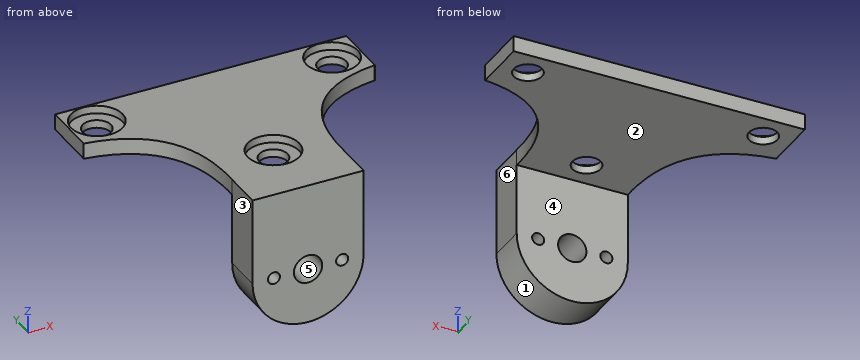
from build123d import *

# Parameters (mm, degrees)
ESQUISSE1_R             = 3.575
BOSS_EXTRU_1_DEPTH      = 4
ESQUISSE17_R            = 6.5
ENL_V_MAT_EXTRU_9_DEPTH = 2
ESQUISSE18_R            = 3.575
ESQUISSE18_R_2          = 1.525
BOSS_EXTRU_6_DEPTH      = 10


with BuildPart() as part:
    # Esquisse1 → Boss.-Extru.1 (new body)
    with BuildSketch(Plane.XY):
        with BuildLine():
            Line((0, 42.932447878), (0, 28.932447878))
            add(Edge.make_bspline(
                [(0, 28.932447878), (23.217449625, 26.022104371), (22.625, 0)],
                knots=[0, 0, 0, 1, 1, 1], degree=2))
            Line((22.625, 0), (36.625, 0))
            Line((36.625, 0), (50.625, 0))
            add(Edge.make_bspline(
                [(73.25, 28.932447878), (50.032550375, 26.022104371), (50.625, 0)],
                knots=[0, 0, 0, 1, 1, 1], degree=2))
            Line((73.25, 28.932447878), (73.4, 28.932447878))
            Line((73.4, 28.932447878), (73.4, 42.932447878))
            Line((73.4, 42.932447878), (0, 42.932447878))
        make_face()
        with Locations((7.025, 36.178525203)):
            Circle(ESQUISSE1_R, mode=Mode.SUBTRACT)
        with Locations((66.375, 36.245920154)):
            Circle(ESQUISSE1_R, mode=Mode.SUBTRACT)
        with Locations((36.625, 7.025)):
            Circle(ESQUISSE1_R, mode=Mode.SUBTRACT)
    extrude(amount=BOSS_EXTRU_1_DEPTH)

    # Esquisse17 → Enlèv. mat.-Extru.9 (cut)
    with BuildSketch(Plane.XY.offset(4)):
        with Locations((7.025, 36.178525203)):
            Circle(ESQUISSE17_R)
        with Locations((66.375, 36.245920154)):
            Circle(ESQUISSE17_R)
        with Locations((36.625, 7.025)):
            Circle(ESQUISSE17_R)
    extrude(amount=-ENL_V_MAT_EXTRU_9_DEPTH, mode=Mode.SUBTRACT)

    # Esquisse18 → Boss.-Extru.6 (add)
    with BuildSketch(Plane.XZ):
        with BuildLine():
            Line((22.625, -18), (22.625, 4))
            Line((22.625, 4), (50.625, 4))
            Line((50.625, 4), (50.625, -18))
            ThreePointArc((50.625, -18), (36.625, -32), (22.625, -18))
        make_face()
        with Locations((36.625, -18)):
            Circle(ESQUISSE18_R, mode=Mode.SUBTRACT)
        with Locations((28.025, -18)):
            Circle(ESQUISSE18_R_2, mode=Mode.SUBTRACT)
        with Locations((45.225, -18)):
            Circle(ESQUISSE18_R_2, mode=Mode.SUBTRACT)
    extrude(amount=BOSS_EXTRU_6_DEPTH)


solid = part.part
Work out the finished part from the listing and answer in its coordinate system (mm). Face numbers are marked on the shaded views. A direction names the side the tool comes from. Round coordinates to 2 decimals unless told otherwise and drop trailing zeros. Write each loop counter-clockwise with the first axis right and the second up, starting at its lowest first coordinate (ties: lowest second). Pieces come first, ordered by that corner, then holes. Notation, with made-up numbers: (30.25, 45.25) - (56.25, 45.25) arc R9 ccw to (56.25, 50.25) - close; hole circle Ø7 at (-3.75, 48.5). An arc over 180 degrees is marked (long way). Answer in a Markdown table with one row per item. Add a question column.
1. Find the intervals of material crossed by line 1 along Z through (x, y) = (63, 27); line 2 along Y through (x, z) = (38, -29); line 3 along X through (y, z) = (-2.5, -18.5), in increasing order. Write a range as from..to.
2. A cutting plane is placed at C-C, the plane z = -1. Determine the outline of the cut face in (x, y) (3 decimals), and give its area (3 significant figures).
3. A cutting plane is placed at A-A, the plane y = 35. Determine the outline of the cut face in (x, z), and give its area (3 significant figures).
4. The mould has two halves that part along X. Classify the marked faces 4, 5 and 6: +X half, -X half, draft (parallel to the pull), parting line (faces both ways), or undercut.
5. Given pin 1 (5 mm diameter, centred on y = -6, z = -2.5, fed in from -X) (3 decimals); pin 2 (8 mm diameter, centred on x = 7.02, y = 36.18, fed in from +Z); pin 3 (5.5 mm diameter, centred on x = 36.625, y = 7.025, fed in from -Z); pin 4 (8 mm diameter, centred on x = 18.5, y = 8.5, fed in from -Z), each flat-ended and moving along its own axis, determine where each tip first touches the part or whether it passes through.
6. For the marked faces 1, 2 and 3, determine the directions among +Z, -Z, +X, -X, +Y, -Y from which every point of the face is accessible in a straight line to the end or side of a thin tool.
7. A cutting plane is placed at B-B, the plane x = 25.5. Determine the outline of the cut face in (y, z), and give its area (3 significant figures).
8. A cutting plane is placed at D-D, the plane z = -25. Determine the outline of the cut face in (x, y).
Worked out:
| question | item | result |
|---|---|---|
| 1 | line 1 | 0..4 |
| 1 | line 2 | -10..0 |
| 1 | line 3 | 22.63..26.58, 29.47..33.09, 40.16..43.78, 46.67..50.62 |
| 2 | outline | (22.625, -10) - (50.625, -10) - (50.625, 0) - (22.625, 0) - close |
| 2 | area | 280 mm^2 |
| 3 | outline | (0, 0) - (3.65, 0) - (3.65, 2) - (0.63, 2) - (0.63, 4) - (0, 4) - close; (10.4, 0) - (63.02, 0) - (63.02, 2) - (60, 2) - (60, 4) - (13.42, 4) - (13.42, 2) - (10.4, 2) - close; (69.73, 0) - (73.4, 0) - (73.4, 4) - (72.75, 4) - (72.75, 2) - (69.73, 2) - close |
| 3 | area | 216 mm^2 |
| 4 | face 4 | draft |
| 4 | face 5 | undercut |
| 4 | face 6 | +X half |
| 5 | pin 1 | x = 22.625 |
| 5 | pin 2 | z = 2 |
| 5 | pin 3 | through |
| 5 | pin 4 | z = 0 |
| 6 | face 1 | -Z, +Y, -Y |
| 6 | face 2 | -Z, +X, -X, +Y |
| 6 | face 3 | +Z, -Z, -X, -Y |
| 7 | outline | (-10, -26.5) - (0, -26.5) - (0, 0) - (42.93, 0) - (42.93, 4) - (-10, 4) - close |
| 7 | area | 477 mm^2 |
| 8 | outline | (24.5, -10) - (48.75, -10) - (48.75, 0) - (24.5, 0) - close |
